from build123d import *

# Parameters (mm, degrees)
F1_DEPTH = 57.15
F2_R     = 6
F3_DEPTH = 25.4


with BuildPart() as f1:
    # F0 (on Top) → F1 (new body)
    with BuildSketch(Plane.XY):
        Polygon((1.104013, -7.248758), (6.829615, -2.668275), (5.725602, 4.580482), (-1.104013, 7.248758), (-6.829615, 2.668275), (-5.725602, -4.580482), align=None)
    extrude(amount=F1_DEPTH)

    # F2 (on Top) → F3 (join)
    with BuildSketch(Plane.XY):
        Circle(F2_R)
    extrude(amount=-F3_DEPTH)


solid = f1.part
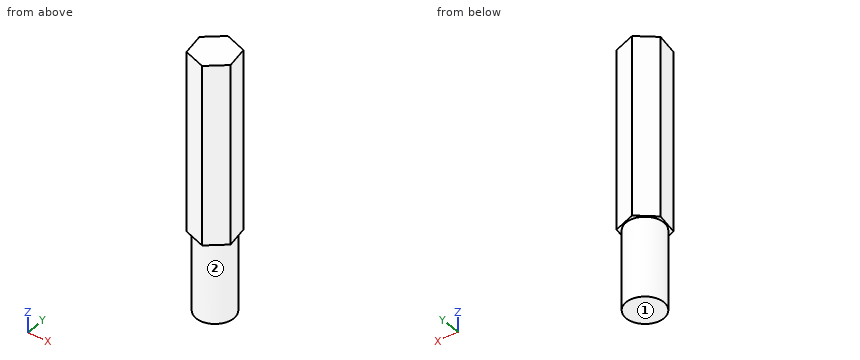
CAD build for the part. Positions are in the model's coordinates, mm. Face numbers are marked on the shaded views. A direction names the side the tool comes from. Give positions to 0.01 mm unless a question says otherwise; leave off trailing zeros. Order: outer loops, then holes, each group sorted by start corner. A loop starts at its lowest first (then second) coordinate and runs counter-clockwise, first axis right, second up. Notation, with made-up numbers: (20.25, -35.75) -> (28.25, -35.75) arc R20 cw to (28.25, -25.75) -> close; hole circle Ø6 at (-37.5, 76). An arc over 180 degrees is marked (long way). Return JSON: item names as keys, results as strings.
Q1. Saw through at A-A (z = -8). Write the cut outline in (x, y).
Working result:
{"outline": "circle Ø12 at (0, 0)"}
Q2. Saw through at C-C (y = 1). Write the cut outline in (x, z).
Working result:
{"outline": "(-6.58, 0) -> (-5.92, 0) -> (-5.92, -25.4) -> (5.92, -25.4) -> (5.92, 0) -> (6.27, 0) -> (6.27, 57.15) -> (-6.58, 57.15) -> close"}
Q3. Saw through at B-B (x = 3). Write the cut outline in (y, z), then the cut area to 3 significant figures.
Working result:
{"outline": "(-5.73, 0) -> (-5.2, 0) -> (-5.2, -25.4) -> (5.2, -25.4) -> (5.2, 0) -> (5.65, 0) -> (5.65, 57.15) -> (-5.73, 57.15) -> close", "area": "914 mm²"}
Q4. Drill centre lines: line 1 (Z direction, x = -2, y = 6.25); line 2 (X direction, y = 1, z = 5.5); line 3 (Y direction, x = 5.5, z = 37.5). Where is each one in solid material? Low to high.
Working result:
{"line 1": "0 to 57.15", "line 2": "-6.58 to 6.27", "line 3": "-3.73 to 4.67"}
Q5. Saw through at D-D (z = 15.5). Write the cut outline in (x, y).
Working result:
{"outline": "(-6.83, 2.67) -> (-5.73, -4.58) -> (1.1, -7.25) -> (6.83, -2.67) -> (5.73, 4.58) -> (-1.1, 7.25) -> close"}
Q6. Flat gauge pins, fed straight in: pin 1 (2 mm diameter, centred on y = -4.5, z = 43.5, fed in from +X); pin 2 (3 mm diameter, centred on x = -3, y = 5.5, fed in from -Z); pin 3 (1.5 mm diameter, centred on x = -1, z = -4.5, fed in from +Y). Where does each tip first touch, or does it go through?
Working result:
{"pin 1": "x = 5.79", "pin 2": "z = -25.4", "pin 3": "y = 5.99"}
Q7. Which spindle directions (+Z, -Z, +X, -X, +Y, -Y) get a long thin tool onto all of the face, cutting with end or side? Do the marked faces 1 and 2. Say none if no direction does.
Working result:
{"face 1": "-Z, +X, -X, +Y, -Y", "face 2": "-Z"}
